The model under review builds one solid part; all positions refer to its coordinate system, in mm. Face numbers are marked on the shaded views. A direction names the side the tool comes from. Coordinates: 2 decimals unless noted, no trailing zeros. Order: outer loops, then holes, each group sorted by start corner. A loop starts at its lowest first (then second) coordinate and runs counter-clockwise, first axis right, second up. Notation, with made-up numbers: M 23.25,24.25 L 63.25,24.25 A21 ccw 63.25,43.25 Z; hole C 76.5,-7 d7. An arc over 180 degrees is marked long. Answer as CSV lines item,"result". Start each with the question number.
Q1. Wall thickness on L1, parallel to Y at x = 0, z = -0.9; L2, parallel to Y at x = 0, z = 0.45; L3, parallel to X at y = 4.75, z = -1.35: over which ranges is each line inside the solid? List them lowest first. Write a range as [from, to].
Q2. For P1, Ø1, axis at x = -5.5, y = 4, coming from the +Z side; P2, Ø1, axis at x = 2, z = -4.5, coming from the -Y side; P3, Ø3, axis at x = 6.5, z = -3.5, coming from the -Y side, all flat-tipped, find the tip position at first contact; note any pin that passes through.
Q3. Consider section C-C on z = -1.8. Write out the cut boundary in (x, y).
Q4. Machinability: for the marked faces 1 and 2, which of the approach directions +Z, -Z, +X, -X, +Y, -Y give a long, thin tool a straight path to every point of the face, cutting with its end or side? Answer none if there is none.
Q5. Consider section A-A on y = 0. Write out the cut boundary in (x, z), and give its area (3 significant figures).
Q6. The part is to be moulded in two halves that separate along X. For the marked faces 3, 4 and 5, say which applies: +X half, -X half, draft (parallel to the pull), parting line (faces both ways), or undercut.
Q7. Consider section D-D on z = 0.45. Write out the cut boundary in (x, y), and give its area (3 significant figures).
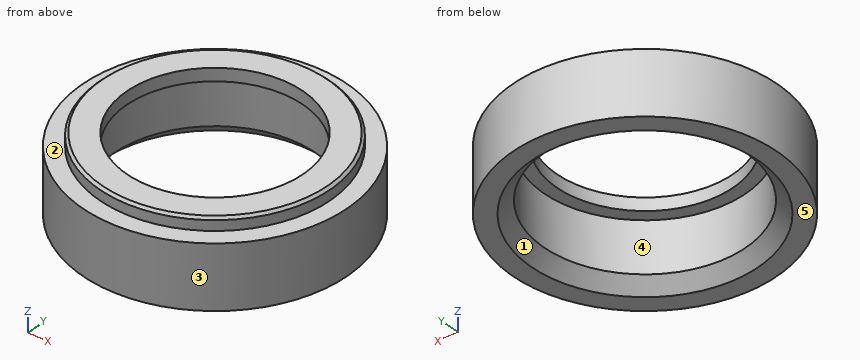
from build123d import *

# Parameters (mm, degrees)
SKETCH_R        = 9.15
PAD_DEPTH       = 1
SKETCH001_R     = 10.5
SKETCH001_R_2   = 8
PAD001_DEPTH    = 5
SKETCH002_R     = 7
POCKET_DEPTH    = 1.001
CHAMFER_SIZE    = 1
CHAMFER001_SIZE = 0.2


with BuildPart() as part:
    # Sketch → Pad (new body)
    with BuildSketch(Plane.XY):
        Circle(SKETCH_R)
    extrude(amount=PAD_DEPTH)

    # Sketch001 → Pad001 (join)
    with BuildSketch(Plane.XY):
        Circle(SKETCH001_R)
        Circle(SKETCH001_R_2, mode=Mode.SUBTRACT)
    extrude(amount=-PAD001_DEPTH)

    # Sketch002 (on Face7 of Pad001) → Pocket (cut, through all)
    with BuildSketch(Plane(origin=(0, 0, 0), x_dir=(1, 0, 0), z_dir=(0, 0, -1))):
        Circle(SKETCH002_R)
    extrude(amount=-POCKET_DEPTH, mode=Mode.SUBTRACT)

    # Chamfer
    chamfer_edges = [part.edges().sort_by_distance(p)[0] for p in [
        (-8, 0, -5),
    ]]
    chamfer(chamfer_edges, length=CHAMFER_SIZE)

    # Chamfer001
    chamfer001_edges = [part.edges().sort_by_distance(p)[0] for p in [
        (-9.15, 0, 1),
    ]]
    chamfer(chamfer001_edges, length=CHAMFER001_SIZE)


solid = part.part
Evaluation:
1,L1,"y = [-10.5, -8], [8, 10.5]"
1,L2,"y = [-9.15, -7], [7, 9.15]"
1,L3,"x = [-9.36, -6.44], [6.44, 9.36]"
2,P1,"stops at z = 1"
2,P2,"stops at y = -10.39"
2,P3,"stops at y = -9.23"
3,outline,"C 0,0 d21; hole C 0,0 d16"
4,face 1,"-Z"
4,face 2,"+Z"
5,outline,"M -10.5,-5 L -9,-5 L -8,-4 L -8,0 L -7,0 L -7,1 L -8.95,1 L -9.15,0.8 L -9.15,0 L -10.5,0 Z; M 7,0 L 8,0 L 8,-4 L 9,-5 L 10.5,-5 L 10.5,0 L 9.15,0 L 9.15,0.8 L 8.95,1 L 7,1 Z"
5,area,"28.3 mm²"
6,face 3,"parting line"
6,face 4,"undercut"
6,face 5,"draft"
7,outline,"C 0,0 d18.3; hole C 0,0 d14"
7,area,"109 mm²"
